from build123d import *

# Parameters (mm, degrees)
BOSS_EXTRUDE1_DEPTH        = 6.35
SKETCH2_R                  = 5.357812451
BOSS_EXTRUDE2_DEPTH        = 6.35
F_10_CLEARANCE_HOLE1_D     = 5
F_10_CLEARANCE_HOLE1_DEPTH = 12.7
SKETCH5_W                  = 2.0193
SKETCH5_H                  = 5.66348411


with BuildPart() as part:
    # Sketch1 → Boss-Extrude1 (new body)
    with BuildSketch(Plane(origin=(0, 0, -3.175), x_dir=(-1, 0, 0), z_dir=(0, 0, -1))):
        with BuildLine():
            Line((-4.475719216, 2.94518093), (-6.469475121, 3.032230191))
            Line((-6.469475121, 3.032230191), (-6.718720366, 2.430498941))
            Line((-6.718720366, 2.430498941), (-5.247368905, 1.082253729))
            ThreePointArc((-5.247368905, 1.082253729), (-5.25486353, 1.045257315), (-5.262097316, 1.008209016))
            Line((-5.262097316, 1.008209016), (-7.137399981, 0.325654666))
            Line((-7.137399981, 0.325654666), (-7.137399981, -0.325654551))
            Line((-7.137399981, -0.325654551), (-5.262097381, -1.008208899))
            ThreePointArc((-5.262097381, -1.008208899), (-5.254863555, -1.045257412), (-5.247368888, -1.08225404))
            Line((-5.247368888, -1.08225404), (-6.718720366, -2.43049927))
            Line((-6.718720366, -2.43049927), (-6.469475121, -3.03223052))
            Line((-6.469475121, -3.03223052), (-4.475719151, -2.945181254))
            ThreePointArc((-4.475719151, -2.945181254), (-4.454858201, -2.97664122), (-4.433776122, -3.007953433))
            Line((-4.433776122, -3.007953433), (-5.277176571, -4.816631533))
            Line((-5.277176571, -4.816631533), (-4.816631353, -5.277176632))
            Line((-4.816631353, -5.277176632), (-3.007953331, -4.433776241))
            ThreePointArc((-3.007953331, -4.433776241), (-2.976641072, -4.454858352), (-2.945181059, -4.475719332))
            Line((-2.945181059, -4.475719332), (-3.032230324, -6.469475317))
            Line((-3.032230324, -6.469475317), (-2.430499074, -6.718720562))
            Line((-2.430499074, -6.718720562), (-1.082253821, -5.247369057))
            ThreePointArc((-1.082253821, -5.247369057), (-1.045257355, -5.254863691), (-1.008209005, -5.262097487))
            Line((-1.008209005, -5.262097487), (-0.325654634, -7.137400208))
            Line((-0.325654634, -7.137400208), (0.325654583, -7.137400208))
            Line((0.325654583, -7.137400208), (1.008208941, -5.262097516))
            ThreePointArc((1.008208941, -5.262097516), (1.045257356, -5.254863709), (1.082253886, -5.247369061))
            Line((1.082253886, -5.247369061), (2.430499137, -6.718720562))
            Line((2.430499137, -6.718720562), (3.032230387, -6.469475317))
            Line((3.032230387, -6.469475317), (2.945181121, -4.475719349))
            ThreePointArc((2.945181121, -4.475719349), (2.976641089, -4.454858399), (3.007953303, -4.433776319))
            Line((3.007953303, -4.433776319), (4.8166314, -5.277176767))
            Line((4.8166314, -5.277176767), (5.277176499, -4.816631549))
            Line((5.277176499, -4.816631549), (4.433776123, -3.007953559))
            ThreePointArc((4.433776123, -3.007953559), (4.454858245, -2.976641285), (4.475719236, -2.945181257))
            Line((4.475719236, -2.945181257), (6.469475184, -3.03223052))
            Line((6.469475184, -3.03223052), (6.718720429, -2.43049927))
            Line((6.718720429, -2.43049927), (5.247368971, -1.08225406))
            ThreePointArc((5.247368971, -1.08225406), (5.254863613, -1.045257562), (5.262097415, -1.008209179))
            Line((5.262097415, -1.008209179), (7.137400075, -0.32565483))
            Line((7.137400075, -0.32565483), (7.137400075, 0.325654387))
            Line((7.137400075, 0.325654387), (5.26209746, 1.008208717))
            ThreePointArc((5.26209746, 1.008208717), (5.254863645, 1.045257174), (5.247368989, 1.082253746))
            Line((5.247368989, 1.082253746), (6.718720429, 2.430498941))
            Line((6.718720429, 2.430498941), (6.469475184, 3.032230191))
            Line((6.469475184, 3.032230191), (4.475719304, 2.945180929))
            ThreePointArc((4.475719304, 2.945180929), (4.454858329, 2.976640935), (4.433776224, 3.007953186))
            Line((4.433776224, 3.007953186), (5.277176634, 4.816631204))
            Line((5.277176634, 4.816631204), (4.816631416, 5.277176303))
            Line((4.816631416, 5.277176303), (3.007953499, 4.433775961))
            ThreePointArc((3.007953499, 4.433775961), (2.976641191, 4.454858106), (2.945181127, 4.47571912))
            Line((2.945181127, 4.47571912), (3.032230387, 6.469474988))
            Line((3.032230387, 6.469474988), (2.430499137, 6.718720233))
            Line((2.430499137, 6.718720233), (1.082253963, 5.24736882))
            ThreePointArc((1.082253963, 5.24736882), (1.045257437, 5.254863468), (1.008209026, 5.262097275))
            Line((1.008209026, 5.262097275), (0.325654697, 7.137399816))
            Line((0.325654697, 7.137399816), (-0.32565452, 7.137399816))
            Line((-0.32565452, 7.137399816), (-1.008208848, 5.262097292))
            ThreePointArc((-1.008208848, 5.262097292), (-1.045257316, 5.254863474), (-1.082253899, 5.247368816))
            Line((-1.082253899, 5.247368816), (-2.430499074, 6.718720233))
            Line((-2.430499074, 6.718720233), (-3.032230324, 6.469474988))
            Line((-3.032230324, 6.469474988), (-2.945181062, 4.475719106))
            ThreePointArc((-2.945181062, 4.475719106), (-2.976641066, 4.454858131), (-3.007953316, 4.433776026))
            Line((-3.007953316, 4.433776026), (-4.816631337, 5.277176438))
            Line((-4.816631337, 5.277176438), (-5.277176436, 4.81663122))
            Line((-5.277176436, 4.81663122), (-4.433776079, 3.007953271))
            ThreePointArc((-4.433776079, 3.007953271), (-4.454858213, 2.976640978), (-4.475719216, 2.94518093))
        make_face()
    extrude(amount=-BOSS_EXTRUDE1_DEPTH)

    # Sketch2 → Boss-Extrude2 (add)
    with BuildSketch(Plane.XY.offset(3.175)):
        with Locations((-1.2e-08, 5.2e-08)):
            Circle(SKETCH2_R)
    extrude(amount=BOSS_EXTRUDE2_DEPTH)

    # #10 Clearance Hole1
    with Locations(Plane.XY.offset(9.525)):
        with Locations((0, 0)):
            Hole(F_10_CLEARANCE_HOLE1_D / 2, depth=F_10_CLEARANCE_HOLE1_DEPTH)

    # Sketch5 → #21 (0.159) Diameter Hole1 (revolve, cut)
    with BuildSketch(Plane(origin=(0, 1.473915707, 6.35), x_dir=(0, 0, -1), z_dir=(1, 0, 0))):
        with Locations((1.00965, 2.831742055)):
            Rectangle(SKETCH5_W, SKETCH5_H)
    revolve(axis=Axis((0, -4.876084293, 6.35), (0, 1, 0)), mode=Mode.SUBTRACT)


solid = part.part
Design review of the part built by this model. Coordinates are the model's own, in mm. A direction names the side the tool comes from. Round coordinates to 2 decimals unless told otherwise and drop trailing zeros. Loops run counter-clockwise (first coordinate to the right, second up) from the corner with the lowest first, then second, coordinate; pieces in that order, holes last. Notation, with made-up numbers: (67.5, -22.5) - (78.5, -22.5) arc R26 cw to (78.5, -4.5) - close; hole circle Ø6 at (-11.75, 31.5). An arc over 180 degrees is marked (long way). One line per item, written item: value. Start each with the question number.
1) Consider section B-B on x = 0. Give the boundary of the cut face in (y, z) (3 decimals), then the cut area to 3 significant figures.
2) Consider section D-D on x = -6. Give the boundary of the cut face in (y, z) (3 decimals).
3) To check wall thickness, follow L1, parallel to Z at x = 0, y = 4.3 (3 decimals); L2, parallel to Y at x = 5.5, z = 0; L3, parallel to Y at x = -6.25, z = -2. State the ranges of each line that lie inside material, in increasing order. Write a range as from..to.
4) Draft analysis for pull direction Y (two halves, no side actions). For faces 1 (the flat face through (-1.747, -5.973, -0.044)), 2 (the cylindrical face through (-1.36, 3.44, 7.84)), 3 (the flat face through (-6.19, -0.67, -0.04)), state which applies: +Y half, -Y half, draft (parallel to the pull), parting line (faces both ways), or undercut.
5) For faces 4 (the flat face through (-6, -2, 3.175)), 5 (the flat face through (1.766, -5.993, -0.044)), 6 (the flat face through (5.973, -1.747, -0.044)), 7 (the flat face through (5.49, -2.99, -0.04)), 8 (the flat face through (2, -6, 3.175)), list the 3-axis set-ups (+Z, -Z, +X, -X, +Y, -Y) from which the entire face can be reached by the end or side of a thin tool; tool diameter is ignored.
6) Consider section A-A on y = 0. Give the boundary of the cut face in (x, z) (3 decimals), then the cut area to 3 significant figures.
7) Consider section C-C on z = 3.5. Give the boundary of the cut face in (x, y).
8) Insertion check: pin 1 Ø3.5 at (x, z) = (0, 6.35) entering from -Y; pin 2 Ø0.6 at (x, y) = (6, 2.5) entering from +Z (3 decimals); pin 3 Ø4 at (x, z) = (4.5, -1) entering from +Y. Each pin has a flat end and moves straight along its axis. Give the tip position at first contact, or say it passes through.
Reported:
1. outline: (-7.137, -3.175) - (-2.5, -3.175) - (-2.5, 9.525) - (-5.358, 9.525) - (-5.358, 3.175) - (-7.137, 3.175) - close; (2.5, -3.175) - (7.137, -3.175) - (7.137, 3.175) - (5.358, 3.175) - (5.358, 4.331) - (2.5, 4.331) - close; (2.5, 8.369) - (5.358, 8.369) - (5.358, 9.525) - (2.5, 9.525) - close
1. area: 83.6 mm^2
2. outline: (-3.012, -3.175) - (-1.772, -3.175) - (-1.772, 3.175) - (-3.012, 3.175) - close; (-0.74, -3.175) - (0.74, -3.175) - (0.74, 3.175) - (-0.74, 3.175) - close; (1.772, -3.175) - (3.012, -3.175) - (3.012, 3.175) - (1.772, 3.175) - close
3. L1: z = -3.175..4.331, 8.369..9.525
3. L2: y = -2.99..-1.31, -0.92..0.92, 1.31..2.99
3. L3: y = -3.02..-2, -0.65..0.65, 2..3.02
4. face 1: -Y half
4. face 2: draft
4. face 3: undercut
5. face 4: +Z, -X, -Y
5. face 5: +Z, -Z, -Y
5. face 6: +Z, -Z, +X
5. face 7: +Z, -Z
5. face 8: +Z, +X, -Y
6. outline: (-7.137, -3.175) - (-2.5, -3.175) - (-2.5, 9.525) - (-5.358, 9.525) - (-5.358, 3.175) - (-7.137, 3.175) - close; (2.5, -3.175) - (7.137, -3.175) - (7.137, 3.175) - (5.358, 3.175) - (5.358, 9.525) - (2.5, 9.525) - close
6. area: 95.2 mm^2
7. outline: circle Ø10.72 at (0, 0); hole circle Ø5 at (0, 0)
8. pin 1: stops at y = -5.36
8. pin 2: stops at z = 3.175
8. pin 3: stops at y = 6.69
